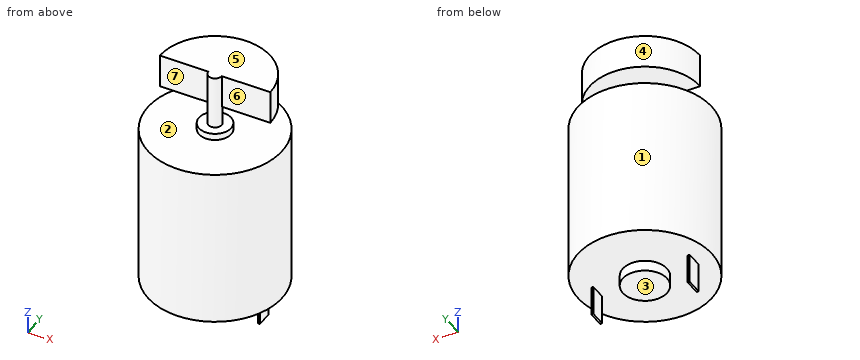
from build123d import *

# Parameters (mm, degrees)
SKETCH1_R           = 12.7
BOSS_EXTRUDE1_DEPTH = 15.24
SKETCH2_R           = 3.048
BOSS_EXTRUDE2_DEPTH = 1.27
SKETCH3_R           = 1.27
BOSS_EXTRUDE3_DEPTH = 10.16
BOSS_EXTRUDE4_DEPTH = 6.35
SKETCH5_R           = 4.191
BOSS_EXTRUDE5_DEPTH = 2.032
SKETCH6_W           = 0.381
SKETCH6_H           = 3.048
BOSS_EXTRUDE6_DEPTH = 5.588


with BuildPart() as part:
    # Sketch1 → Boss-Extrude1 (new, symmetric)
    with BuildSketch(Plane.XY):
        with Locations(Location((0, 0, 0), (0, 0, 180))):
            Circle(SKETCH1_R)
    extrude(amount=BOSS_EXTRUDE1_DEPTH, both=True)

    # Sketch2 → Boss-Extrude2 (add)
    with BuildSketch(Plane.XY.offset(15.24)):
        Circle(SKETCH2_R)
    extrude(amount=BOSS_EXTRUDE2_DEPTH)

    # Sketch3 → Boss-Extrude3 (add)
    with BuildSketch(Plane.XY.offset(16.51)):
        Circle(SKETCH3_R)
    extrude(amount=BOSS_EXTRUDE3_DEPTH)

    # Sketch4 → Boss-Extrude4 (add)
    with BuildSketch(Plane.XY.offset(26.67)):
        with BuildLine():
            Line((-10.4775, 0), (10.4775, 0))
            ThreePointArc((10.4775, 0), (0, 10.4775), (-10.4775, 0))
        make_face()
    extrude(amount=-BOSS_EXTRUDE4_DEPTH)

    # Sketch5 → Boss-Extrude5 (add)
    with BuildSketch(Plane(origin=(0, 0, -15.24), x_dir=(-1, 0, 0), z_dir=(0, 0, -1))):
        Circle(SKETCH5_R)
    extrude(amount=BOSS_EXTRUDE5_DEPTH)

    # Sketch6 → Boss-Extrude6 (add)
    with BuildSketch(Plane(origin=(0, 0, -15.24), x_dir=(-1, 0, 0), z_dir=(0, 0, -1))):
        with Locations((-9.144, 0)):
            Rectangle(SKETCH6_W, SKETCH6_H)
    boss_extrude6 = extrude(amount=BOSS_EXTRUDE6_DEPTH)

    # Mirror1: Boss-Extrude6 across plane
    add(boss_extrude6.mirror(Plane(origin=(0, 0, 0), x_dir=(0, 0, 1), z_dir=(1, 0, 0))))


solid = part.part
Source: CAD feature listing. Evaluate the final solid. Frame: model axes, mm. Face numbers are marked on the shaded views. A direction names the side the tool comes from. Give positions to 0.01 mm unless a question says otherwise; leave off trailing zeros. Write each loop counter-clockwise with the first axis right and the second up, starting at its lowest first coordinate (ties: lowest second). Pieces come first, ordered by that corner, then holes. Notation, with made-up numbers: M 86.25,20.5 L 90.25,20.5 A9 ccw 90.25,31.5 Z; hole C 18.5,60 d9. An arc over 180 degrees is marked long. Return JSON: item names as keys, results as strings. Group by question number.
1) Cut plane A-A, the plane z = -18. Output: boundary loops of the cut face in (x, y).
2) Material intervals for line 1 along Z through (x, y) = (0.25, 3.25); line 2 along Z through (x, y) = (7.5, -4.75); line 3 along Z through (x, y) = (-2.75, -0.25), sorted ascending. Write a range as [from, to].
3) Set-up query: the marked faces 4, 5, 6 and 7. Return all of +Z, -Z, +X, -X, +Y, -Y with unobstructed straight access to the full face (end or side cutting, diameter ignored); none if empty.
4) Cut plane C-C, the plane x = 0. Output: boundary loops of the cut face in (y, z), plus the area to 3 significant figures.
5) Cut plane B-B, the plane x = 6.5. Output: boundary loops of the cut face in (y, z), plus the area to 3 significant figures.
6) Pull-direction query (Z, two-part tool) for the marked faces 1, 2 and 3; classes: pulls with the +Z half, pulls with the -Z half, needs draft (parallel to the pull), parting line crosses it, or undercut.
7) Pin query (flat end, axial travel): P1, Ø7, axis at x = -7.5, z = 23.5, coming from the -Y side; P2, Ø6, axis at x = -6, z = 0, coming from the +Y side; P3, Ø4, axis at x = 1, y = 0, coming from the -Z side. Return the tip coordinate at first contact, or that it passes through.
8) Cut plane D-D, the plane y = 0.5. Output: boundary loops of the cut face in (x, z).
Recorded:
{
 "1": {"outline": "M -9.33,-1.52 L -8.95,-1.52 L -8.95,1.52 L -9.33,1.52 Z; M 8.95,-1.52 L 9.33,-1.52 L 9.33,1.52 L 8.95,1.52 Z"},
 "2": {"line 1": "z = [-17.27, 15.24], [20.32, 26.67]", "line 2": "z = [-15.24, 15.24]", "line 3": "z = [-17.27, 16.51]"},
 "3": {"face 4": "+Z, +Y", "face 5": "+Z, +X, -X, +Y, -Y", "face 6": "+Z, +X, -Y", "face 7": "+Z, -X, -Y"},
 "4": {"outline": "M -12.7,-15.24 L -4.19,-15.24 L -4.19,-17.27 L 4.19,-17.27 L 4.19,-15.24 L 12.7,-15.24 L 12.7,15.24 L 3.05,15.24 L 3.05,16.51 L 1.27,16.51 L 1.27,20.32 L 10.48,20.32 L 10.48,26.67 L -1.27,26.67 L -1.27,16.51 L -3.05,16.51 L -3.05,15.24 L -12.7,15.24 Z", "area": "883 mm²"},
 "5": {"outline": "M -10.91,-15.24 L 10.91,-15.24 L 10.91,15.24 L -10.91,15.24 Z; M 0,20.32 L 8.22,20.32 L 8.22,26.67 L 0,26.67 Z", "area": "717 mm²"},
 "6": {"face 1": "needs draft", "face 2": "undercut", "face 3": "pulls with the -Z half"},
 "7": {"P1": "stops at y = 0", "P2": "stops at y = 12.34", "P3": "stops at z = -17.27"},
 "8": {"outline": "M -12.69,-15.24 L -9.33,-15.24 L -9.33,-20.83 L -8.95,-20.83 L -8.95,-15.24 L -4.16,-15.24 L -4.16,-17.27 L 4.16,-17.27 L 4.16,-15.24 L 8.95,-15.24 L 8.95,-20.83 L 9.33,-20.83 L 9.33,-15.24 L 12.69,-15.24 L 12.69,15.24 L 3.01,15.24 L 3.01,16.51 L 1.17,16.51 L 1.17,20.32 L 10.47,20.32 L 10.47,26.67 L -10.47,26.67 L -10.47,20.32 L -1.17,20.32 L -1.17,16.51 L -3.01,16.51 L -3.01,15.24 L -12.69,15.24 Z"}
}
